Input: part model. Units: mm. Frame: model coordinates. Face numbers are marked on the shaded views. A direction names the side the tool comes from. Round coordinates to 2 decimals unless told otherwise and drop trailing zeros. Order: outer loops, then holes, each group sorted by start corner. A loop starts at its lowest first (then second) coordinate and runs counter-clockwise, first axis right, second up. Notation, with made-up numbers: (8.5, 15) -> (56.5, 15) arc R7 ccw to (56.5, 19) -> close; hole circle Ø6 at (74.25, 69). An arc over 180 degrees is marked (long way). Answer as CSV lines item,"result". Start each with the question number.
1) Access query for the marked faces 1, 2 and 3. Directions: +Z, -Z, +X, -X, +Y, -Y. A direction counts if a zero-diameter tool reaches every point of the face in a straight line with its end or side. Return the directions, or none.
2) Section query A-A, the plane z = -3.5. Output: boundary loops of the cut face in (x, y).
3) Line query: L1, parallel to Y at x = 0, z = 76; L2, parallel to Y at x = 0, z = 29; L3, parallel to Z at x = -14, y = 11. Output: solid intervals per line, ascending.
4) Section query B-B, the plane z = 19. Output: boundary loops of the cut face in (x, y), and give its area (3 significant figures).
5) First-contact query: P1, Ø10, axis at y = 15.5, z = 18, coming from the -X side; P2, Ø8, axis at y = 7, z = -2, coming from the +X side; P3, Ø1.5, axis at x = 0, y = 19, coming from the +Z side. Flat tips, straight axial feed; report the tip coordinate or a pass-through.
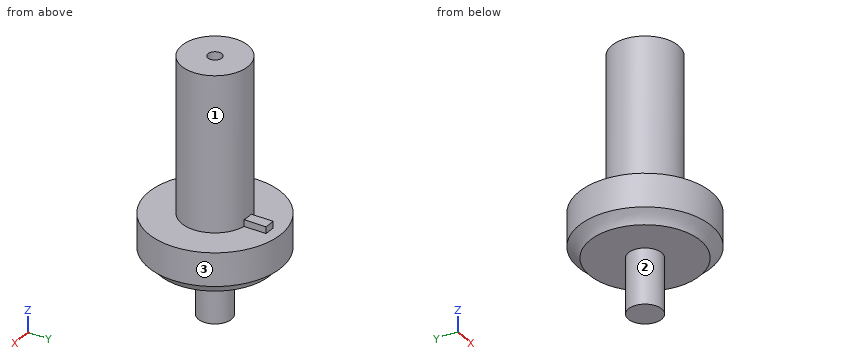
```python
from build123d import *

# Parameters (mm, degrees)
SKETCH1_R           = 15
BOSS_EXTRUDE1_DEPTH = 80
SKETCH1_2_R         = 15
SKETCH2_R           = 25
SKETCH3_R           = 7.5
BOSS_EXTRUDE2_DEPTH = 25
SKETCH4_W           = 5
SKETCH4_H           = 25
BOSS_EXTRUDE3_DEPTH = 3
SKETCH5_R           = 3.15
CUT_EXTRUDE1_DEPTH  = 6
SKETCH6_R           = 30
BOSS_EXTRUDE4_DEPTH = 15


with BuildPart() as part:
    # Sketch1 → Boss-Extrude1 (new body)
    with BuildSketch(Plane.XY):
        Circle(SKETCH1_R)
    extrude(amount=BOSS_EXTRUDE1_DEPTH)

    # Sketch1<2> → Loft1 section 0
    with BuildSketch(Plane.XY):
        Circle(SKETCH1_2_R)
    # Sketch2 → Loft1 section 1
    with BuildSketch(Plane(origin=(0, 0, -10), x_dir=(-1, 0, 0), z_dir=(0, 0, -1))):
        Circle(SKETCH2_R)
    loft()

    # Sketch3 → Boss-Extrude2 (add)
    with BuildSketch(Plane(origin=(0, 0, -10), x_dir=(-1, 0, 0), z_dir=(0, 0, -1))):
        Circle(SKETCH3_R)
    extrude(amount=BOSS_EXTRUDE2_DEPTH)

    # Sketch4 → Boss-Extrude3 (add)
    with BuildSketch(Plane.XY.offset(10)):
        with Locations((0.003158662, 12.374368268)):
            Rectangle(SKETCH4_W, SKETCH4_H)
    extrude(amount=BOSS_EXTRUDE3_DEPTH)

    # Sketch5 → Cut-Extrude1 (cut)
    with BuildSketch(Plane.XY.offset(80)):
        Circle(SKETCH5_R)
    extrude(amount=-CUT_EXTRUDE1_DEPTH, mode=Mode.SUBTRACT)

    # Sketch6 → Boss-Extrude4 (add)
    with BuildSketch(Plane.XY.offset(10)):
        Circle(SKETCH6_R)
    extrude(amount=-BOSS_EXTRUDE4_DEPTH)

    # Loft3: read off the stored shape, not the designer's step
    # Loft3: loft between two sections, ruled curve by curve
    loft3_from = [
        Edge.make_bspline([(-27.865450574, 11.113805123, -5), (-5.637840328, 66.844706271, -5), (50.09306082, 44.617096025, -5), (27.865450574, -11.113805123, -5), (5.637840328, -66.844706271, -5), (-50.09306082, -44.617096025, -5), (-27.865450574, 11.113805123, -5)], [0, 0, 0, 0, 0.5, 0.5, 0.5, 1, 1, 1, 1], 3, [1, 0.333333333, 0.333333333, 1, 0.333333333, 0.333333333, 1]),
    ]
    loft3_to = [
        Edge.make_bspline([(-16.473801558, 18.804623427, -10), (21.135445295, 51.752226543, -10), (54.083048412, 14.14297969, -10), (16.473801558, -18.804623427, -10), (-21.135445295, -51.752226543, -10), (-54.083048412, -14.14297969, -10), (-16.473801558, 18.804623427, -10)], [0, 0, 0, 0, 0.5, 0.5, 0.5, 1, 1, 1, 1], 3, [1, 0.333333333, 0.333333333, 1, 0.333333333, 0.333333333, 1]),
    ]
    loft3 = Solid(Shell([*[Face.make_surface_from_curves(loft3_from[k], loft3_to[k]) for k in range(1)], Face(Wire(loft3_from)), Face(Wire(loft3_to))]))
    add(loft3)


solid = part.part
```
Findings:
1,face 1,"+Z"
1,face 2,"-Z"
1,face 3,"+Z, -Z"
2,outline,"circle Ø60 at (0, 0)"
3,L1,"y = -15 to -3.15, 3.15 to 15"
3,L2,"y = -15 to 15"
3,L3,"z = -10 to 10"
4,outline,"circle Ø30 at (0, 0)"
4,area,"707 mm^2"
5,P1,"stops at x = -10.71"
5,P2,"stops at x = 29.85"
5,P3,"stops at z = 13"
